Study the drawing (mm; zero at the part's minimum x, y, z) and answer. Coordinates: 2 decimals unless noted, no trailing zeros. Loops run counter-clockwise (first coordinate to the right, second up) from the corner with the lowest first, then second, coordinate; pieces in that order, holes last. Notation, with made-up numbers: (45, 11.5) - (95, 11.5) arc R21 ccw to (95, 50.5) - close; hole circle Ø6 at (-38, -8). An arc over 180 degrees is marked (long way). Use one line per item in the form item = value.
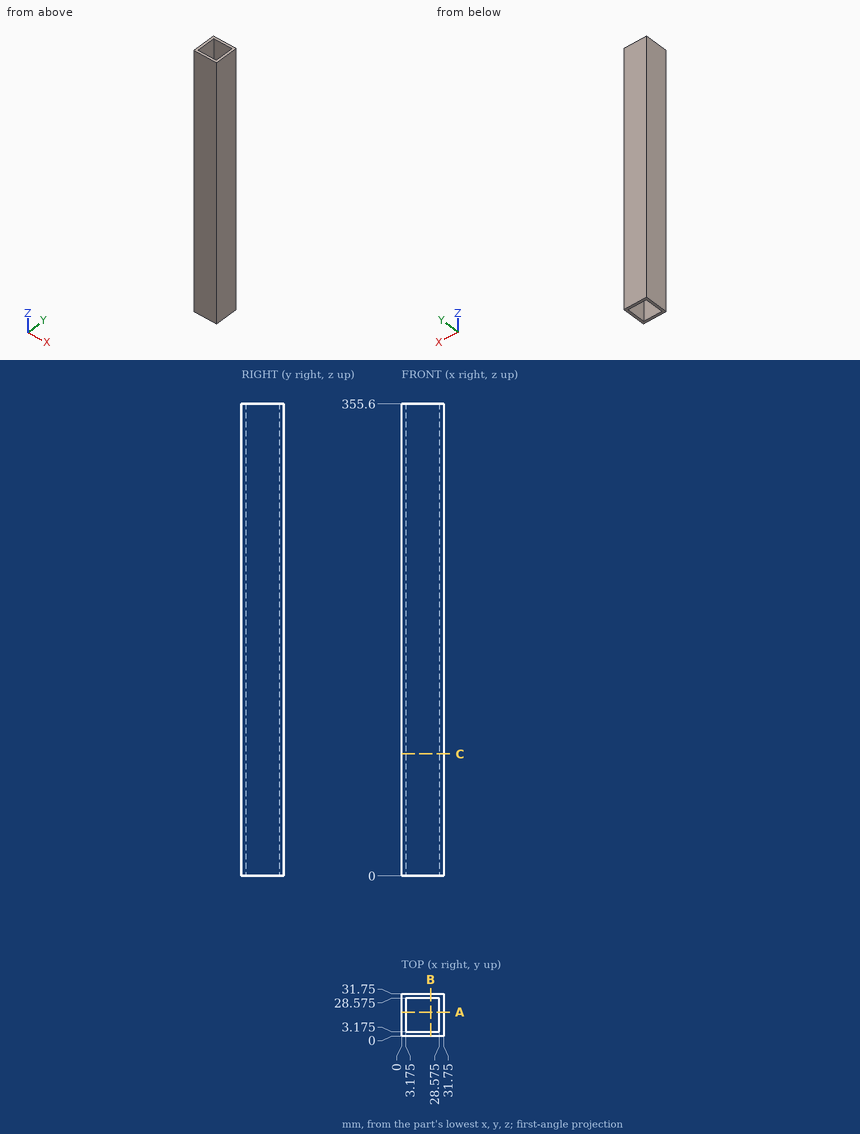
Item 1: Find the intervals of material crossed by L1, parallel to X at y = 14.5, z = 107.5 (3 decimals), in increasing order.
Results below:
L1 = 0 to 3.175, 28.575 to 31.75
Item 2: The part is cut by section A-A on y = 18. Give the vertices of the cut face in (x, z) (3 decimals).
Results below:
outline = (0, 0) - (3.175, 0) - (3.175, 355.6) - (0, 355.6) - close; (28.575, 0) - (31.75, 0) - (31.75, 355.6) - (28.575, 355.6) - close
Item 3: The part is cut by section C-C on z = 92. Give the vertices of the cut face in (x, y) (3 decimals), plus the area to 3 significant figures.
Results below:
outline = (0, 0) - (31.75, 0) - (31.75, 31.75) - (0, 31.75) - close; hole (3.175, 3.175) - (28.575, 3.175) - (28.575, 28.575) - (3.175, 28.575) - close
area = 363 mm²
